The listing builds one solid part. Answer for the finished solid, in the listing's coordinates (mm). Face numbers are marked on the shaded views. A direction names the side the tool comes from. Coordinates: 2 decimals unless noted, no trailing zeros. Order: outer loops, then holes, each group sorted by start corner. A loop starts at its lowest first (then second) coordinate and runs counter-clockwise, first axis right, second up. Notation, with made-up numbers: M -16.5,-17.75 L 12.5,-17.75 A14 cw 12.5,-6.75 Z; hole C -20,-23 d8. An arc over 180 degrees is marked long. One line per item, written item: value. Start each with the question number.
Q1. The part is cut by section B-B on x = 5.08. Give the vertices of the cut face in (y, z).
Q2. The part is cut by section A-A on z = 0. Give the vertices of the cut face in (x, y), then the cut area to 3 significant figures.
Q3. The part is cut by section D-D on x = 8.75. Give the vertices of the cut face in (y, z), then the cut area to 3 significant figures.
Q4. Each of these flat-tipped pins is pushed along its axis until it touches: pin 1 Ø2.5 at (x, z) = (8, 4) entering from -Y; pin 2 Ø1.5 at (y, z) = (5.5, 4) entering from -X; pin 3 Ø4 at (x, y) = (5.5, 2) entering from +Z. Where does it stop, or does it pass through?
Q5. Determine the mould class of the marked faces 4, 5 and 6 for opening direction X: pulls with the +X half, pulls with the -X half, needs draft (parallel to the pull), parting line crosses it, or undercut.
Q6. Straight lines are drawn through the part: line 1 along X through (y, z) = (5, 0); line 2 along X through (y, z) = (8.25, 0); line 3 along Z through (x, y) = (2.5, 2.25). For each, find the intervals that lie inside material, in ascending order. Write a range as [from, to].
Q7. For the marked faces 1, 2 and 3, determine the directions among +Z, -Z, +X, -X, +Y, -Y from which every point of the face is accessible in a straight line to the end or side of a thin tool.
Q8. The part is cut by section C-C on y = 4.75. Give the vertices of the cut face in (x, z).
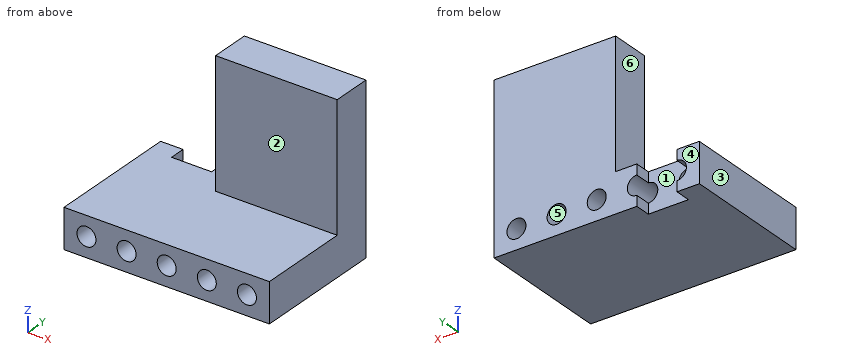
Autodesk Fusion 360 part; units mm, degrees
sketch "Skizze1" plane through (0, 0, 0) normal (0, 1, 0) x (1, 0, 0)
  circle A0 centre (0, 0) radius 0.6
  circle A1 centre (2.54, 0) radius 0.6
  circle A2 centre (5.08, 0) radius 0.6
  circle A3 centre (7.62, 0) radius 0.6
  circle A4 centre (10.16, 0) radius 0.6
  line L0 (11.58, 1.25) -> (-1.42, 1.25)
  line L1 (-1.42, 1.25) -> (-1.42, -1.25)
  line L2 (-1.42, -1.25) -> (11.58, -1.25)
  line L3 (11.58, -1.25) -> (11.58, 1.25)
  line L4 (11.58, 1.25) -> (-1.42, -1.25) construction
  line L5 (-1.42, 1.25) -> (11.58, -1.25) construction
  point P0 (5.08, 0)
  dimension "d1" = 1.2
  dimension "d4" = 2.54
  dimension "d5" = 0
  dimension "d6" = 13
  dimension "d7" = 2.5
extrude "Extrusion1" add sketch "Skizze1" along normal blind 8.4
sketch "Skizze4" plane through (0, 0, 1.25) normal (0, 0, 1) x (1, 0, 0)
  line L0 (-1.42, 0) -> (11.58, 0)
  line L1 (11.58, 0) -> (11.58, 8.4)
  line L2 (11.58, 8.4) -> (-1.42, 8.4)
  line L3 (-1.42, 8.4) -> (-1.42, 0)
  line L4 (11.58, 8.4) -> (3.88, 8.4)
  line L5 (3.88, 8.4) -> (3.88, 5.9)
  line L6 (3.88, 5.9) -> (11.58, 5.9)
  line L7 (11.58, 5.9) -> (11.58, 8.4)
  dimension "d10" = 7.7
  dimension "d11" = 2.5
extrude "Extrusion2" add sketch "Skizze4" along normal blind 8 contours L1 L2 L4 L5 L6 L7
sketch "Skizze5" plane through (0, 8.4, 0) normal (0, 1, 0) x (-1, 0, 0)
  circle A0 centre (-7.62, 0) radius 0.6
  circle A1 centre (-5.08, 0) radius 0.6
  circle A2 centre (-10.16, 0) radius 0.6
  circle A3 centre (-2.54, 0) radius 0.6
  circle A4 centre (0, 0) radius 0.6
  line L0 (-11.58, 9.25) -> (-11.58, -1.25)
  line L1 (-11.58, -1.25) -> (1.42, -1.25)
  line L2 (1.42, -1.25) -> (1.42, 1.25)
  line L3 (1.42, 1.25) -> (-3.88, 1.25)
  line L4 (-3.88, 1.25) -> (-3.88, 9.25)
  line L5 (-3.88, 9.25) -> (-11.58, 9.25)
  line L6 (0, -1.25) -> (-2.54, -1.25)
  line L7 (-2.54, -1.25) -> (-2.54, 1.25)
  line L8 (-2.54, 1.25) -> (0, 1.25)
  line L9 (0, 1.25) -> (0, -1.25)
extrude "Extrusion3" cut sketch "Skizze5" against normal blind 1 contours A3 A4 L1 L3 L6 L7 L8 L9
Output:
1. outline: M 0,-1.25 L 8.4,-1.25 L 8.4,-0.6 L 0,-0.6 Z; M 0,0.6 L 8.4,0.6 L 8.4,9.25 L 5.9,9.25 L 5.9,1.25 L 0,1.25 Z
2. outline: M -1.42,0 L -0.6,0 L -0.6,8.4 L -1.42,8.4 Z; M 0.6,0 L 1.94,0 L 1.94,7.4 L 0.6,7.4 Z; M 3.14,0 L 4.48,0 L 4.48,8.4 L 3.14,8.4 Z; M 5.68,0 L 7.02,0 L 7.02,8.4 L 5.68,8.4 Z; M 8.22,0 L 9.56,0 L 9.56,8.4 L 8.22,8.4 Z; M 10.76,0 L 11.58,0 L 11.58,8.4 L 10.76,8.4 Z
2. area: 57.5 mm^2
3. outline: M 0,-1.25 L 8.4,-1.25 L 8.4,9.25 L 5.9,9.25 L 5.9,1.25 L 0,1.25 Z
3. area: 41.0 mm^2
4. pin 1: stops at y = 5.9
4. pin 2: stops at x = 3.88
4. pin 3: stops at z = 1.25
5. face 4: needs draft
5. face 5: undercut
5. face 6: pulls with the -X half
6. line 1: x = [-1.42, -0.6], [0.6, 1.94], [3.14, 4.48], [5.68, 7.02], [8.22, 9.56], [10.76, 11.58]
6. line 2: x = [-1.42, -0.6], [3.14, 4.48], [5.68, 7.02], [8.22, 9.56], [10.76, 11.58]
6. line 3: z = [-1.25, -0.6], [0.6, 1.25]
7. face 1: +Z, -Z, +Y
7. face 2: +Z, +X, -X, -Y
7. face 3: +Z, -Z, -X, +Y, -Y
8. outline: M -1.42,-1.25 L 11.58,-1.25 L 11.58,1.25 L -1.42,1.25 Z; hole C 0,0 d1.2; hole C 2.54,0 d1.2; hole C 5.08,0 d1.2; hole C 7.62,0 d1.2; hole C 10.16,0 d1.2
